Could you check a few things on this model? Use its own coordinates, in mm. A direction names the side the tool comes from. Give positions to 0.01 mm unless a question says otherwise; leave off trailing zeros. Loops run counter-clockwise (first coordinate to the right, second up) from the corner with the lowest first, then second, coordinate; pieces in that order, holes last. Notation, with made-up numbers: M 14.5,73.25 L 30.5,73.25 A9 ccw 30.5,90.25 Z; hole C 32.5,58.5 d7. An arc over 180 degrees is marked long. Use CSV: the item, a comma, the result in double quotes.
```python
from build123d import *

# Parameters (mm, degrees)
SKETCH015_W     = 20
SKETCH015_H     = 30
PAD006_DEPTH    = 40
SKETCH016_R     = 1.9
POCKET009_DEPTH = 20.001
SKETCH017_R     = 3
POCKET010_DEPTH = 3
SKETCH018_R     = 0.5
POCKET011_DEPTH = 0.5


with BuildPart() as part:
    # Sketch015 → Pad006 (new body)
    with BuildSketch(Plane.XY):
        with Locations((-43, 0)):
            Rectangle(SKETCH015_W, SKETCH015_H)
    extrude(amount=PAD006_DEPTH)

    # Sketch016 (on Face4 of Pad006) → Pocket009 (cut, through all)
    with BuildSketch(Plane(origin=(-53, 0, 0), x_dir=(0, -1, 0), z_dir=(-1, 0, 0))):
        with Locations((-11, 36)):
            Circle(SKETCH016_R)
        with Locations((11, 20)):
            Circle(SKETCH016_R)
        with Locations((-11, 20)):
            Circle(SKETCH016_R)
        with Locations((-11, 4)):
            Circle(SKETCH016_R)
        with Locations((11, 4)):
            Circle(SKETCH016_R)
    extrude(amount=-POCKET009_DEPTH, mode=Mode.SUBTRACT)

    # Sketch017 (on Face2 of Pocket009) → Pocket010 (cut)
    with BuildSketch(Plane(origin=(-53, 0, 0), x_dir=(0, -1, 0), z_dir=(-1, 0, 0))):
        with Locations((-11, 36)):
            Circle(SKETCH017_R)
        with Locations((-11, 20)):
            Circle(SKETCH017_R)
        with Locations((-11, 4)):
            Circle(SKETCH017_R)
        with Locations((11, 4)):
            Circle(SKETCH017_R)
        with Locations((11, 20)):
            Circle(SKETCH017_R)
    extrude(amount=-POCKET010_DEPTH, mode=Mode.SUBTRACT)

    # Sketch018 (on Face5 of Pocket010) → Pocket011 (cut)
    with BuildSketch(Plane.XY.offset(40)):
        with Locations((-43, -4)):
            Circle(SKETCH018_R)
    extrude(amount=-POCKET011_DEPTH, mode=Mode.SUBTRACT)


solid = part.part
```
1. Please list where these lines run through material, in increasing order: line 1 (Z direction, x = -51.4, y = -11); line 2 (Y direction, x = -43, z = 39.8); line 3 (Y direction, x = -48.5, z = 21).
Outcome:
line 1,"0 to 1, 7 to 17, 23 to 40"
line 2,"-15 to -4.5, -3.5 to 15"
line 3,"-15 to -12.62, -9.38 to 9.38, 12.62 to 15"
2. Which directions (+Z, -Z, +X, -X, +Y, -Y) give clear straight access to the entire face, cutting with the end or side of a thin tool? Please do faces 4 (the face through (-51.5, -8.6, 2.2)), 5 (the face through (-43, -4, 39.5)), 6 (the face through (-41.619, -10.753, 21.884)).
Outcome:
face 4,"-X"
face 5,"+Z"
face 6,"+X, -X"
3. If we mould it in two halves opening along Y, with no side actions, what happens to faces 1 (the face through (-51.5, 13.4, 2.2)), 2 (the face through (-43, -15, 20)), 3 (the face through (-53, 0, 20))? For each: +Y half, -Y half, draft (parallel to the pull), parting line (faces both ways), or undercut.
Outcome:
face 1,"undercut"
face 2,"-Y half"
face 3,"draft"
4. I want a section at A-A, the plane z = 4. List the corners of the cut face in (x, y) for me.
Outcome:
outline,"M -53,-15 L -33,-15 L -33,-12.9 L -50,-12.9 L -50,-14 L -53,-14 Z; M -53,-8 L -50,-8 L -50,-9.1 L -33,-9.1 L -33,9.1 L -50,9.1 L -50,8 L -53,8 Z; M -53,14 L -50,14 L -50,12.9 L -33,12.9 L -33,15 L -53,15 Z"
5. I want a section at B-B, the plane x = -48.25. List the corners of the cut face in (y, z) for me.
Outcome:
outline,"M -15,0 L 15,0 L 15,40 L -15,40 Z; hole C -11,4 d3.8; hole C -11,20 d3.8; hole C 11,4 d3.8; hole C 11,20 d3.8; hole C 11,36 d3.8"
6. I want a section at D-D, the plane x = -43. List the corners of the cut face in (y, z) for me.
Outcome:
outline,"M -15,0 L 15,0 L 15,40 L -3.5,40 L -3.5,39.5 L -4.5,39.5 L -4.5,40 L -15,40 Z; hole C -11,4 d3.8; hole C -11,20 d3.8; hole C 11,4 d3.8; hole C 11,20 d3.8; hole C 11,36 d3.8"
7. I want a section at C-C, the plane z = 36. List the corners of the cut face in (x, y) for me, then the cut area to 3 significant figures.
Outcome:
outline,"M -53,-15 L -33,-15 L -33,9.1 L -50,9.1 L -50,8 L -53,8 Z; M -53,14 L -50,14 L -50,12.9 L -33,12.9 L -33,15 L -53,15 Z"
area,"517 mm2"
8. I'm going to push flat-ended pins straight in: pin 1 Ø5 at (y, z) = (11, 4) entering from +X; pin 2 Ø5 at (y, z) = (11, 36) entering from -X; pin 3 Ø0.5 at (x, y) = (-43, -4) entering from +Z. Where does each tip first touch, or does it pass through?
Outcome:
pin 1,"x = -33"
pin 2,"x = -50"
pin 3,"z = 39.5"
